from build123d import *

# Parameters (mm, degrees)
EXTRUDE_1_DEPTH             = 10
CUT_EXTRUDE_1_DEPTH         = 2
CUT_EXTRUDE_2_DEPTH         = 2
SKETCH_4_R                  = 35.00000000000001
CUT_EXTRUDE_3_DEPTH         = 3
CUT_EXTRUDE_4_DEPTH         = 62.016391240387215
HOLE_WIZARD_M3_1_D          = 2.5
HOLE_WIZARD_1_D             = 3.4
HOLE_WIZARD_1_CSINK_D       = 6.6
HOLE_WIZARD_1_CSINK_ANGLE   = 90
SKETCH_11_R                 = 4.000000000000005
SKETCH_11_R_2               = 3.999999999999999
SKETCH_11_R_3               = 4
CUT_EXTRUDE_5_DEPTH         = 1
CHAMFER_1_SIZE              = 10
EXTRUDE_2_DEPTH             = 14
EXTRUDE_2_DIRECTION_2_REACH = 63.628
SKETCH_13_R                 = 1.5000000000000009
SKETCH_13_R_2               = 1.5000000000000042
CUT_EXTRUDE_6_DEPTH         = 8
SKETCH_13_3_R               = 1.5000000000000009
SKETCH_13_3_R_2             = 1.5000000000000042
CUT_EXTRUDE_7_DEPTH         = 3
MIRROR_START                = 45.74011537
MIRROR_6_OUTLINE_R          = 1.5
MIRROR_6_DEPTH              = 5
CUT_EXTRUDE_8_DEPTH         = 83.20937791832523
FILLET_1_R                  = 3
FILLET_2_R                  = 3
FILLET_5_R                  = 3
CHAMFER_2_SIZE              = 0.5


# Read off the part's stored shape, not the designer's step: 镜向6
with BuildPart() as part:
    # 草图1 → 凸台-拉伸1 (new body)
    with BuildSketch(Plane(origin=(0, 0, 0), x_dir=(1, 0, 0), z_dir=(0, 1, 0))):
        Polygon((-43, 43), (42.999999999999986, 43), (43, -42.99999999999999), (-43, -42.99999999999999), align=None)
    extrude(amount=EXTRUDE_1_DEPTH)

    # 草图2 → 切除-拉伸1 (cut)
    with BuildSketch(Plane.XZ):
        Polygon((42.99999999999999, 7.000000000000008), (-43, 7.000000000000008), (-43, -43), (43, -43), align=None)
    extrude(amount=-CUT_EXTRUDE_1_DEPTH, mode=Mode.SUBTRACT)

    # 草图3 → 切除-拉伸2 (cut)
    with BuildSketch(Plane(origin=(0, 10, 0), x_dir=(1, 0, 0), z_dir=(0, 1, 0))):
        with BuildLine():
            Line((-24.686291501015234, -42.99999999999999), (24.686291501015248, -42.999999999999986))
            Line((24.686291501015244, -42.999999999999986), (24.686291501015237, -39.994837315919945))
            ThreePointArc((24.686291501015248, -39.99483731591996), (33.99829514057673, -32.45174768073728), (41.099999999999305, -22.79890348240587))
            Line((41.10000000000001, -22.798903482406033), (41.1, 22.798903482403997))
            ThreePointArc((41.10000000000031, 22.798903482404068), (33.23401871576778, 33.234018715767704), (22.79890348240416, 41.10000000000025))
            Line((22.798903482404093, 41.099999999999994), (-22.798903482403766, 41.099999999999994))
            ThreePointArc((-22.798903482403876, 41.1000000000004), (-33.23401871576702, 33.23401871576845), (-41.099999999999426, 22.798903482405624))
            Line((-41.1, 22.798903482405752), (-41.099999999999994, -22.798903482407027))
            ThreePointArc((-41.09999999999881, -22.798903482406732), (-33.99829514057638, -32.45174768073764), (-24.68629150101524, -39.99483731591995))
            Line((-24.686291501015234, -39.994837315919945), (-24.686291501015234, -42.99999999999999))
        make_face()
    extrude(amount=-CUT_EXTRUDE_2_DEPTH, mode=Mode.SUBTRACT)

    # 草图4 → 切除-拉伸3 (cut)
    with BuildSketch(Plane(origin=(0, 8, 0), x_dir=(1, 0, 0), z_dir=(0, 1, 0))):
        with Locations(Location((0, 0, 0), (0, 0, 270))):
            Circle(SKETCH_4_R)
    extrude(amount=-CUT_EXTRUDE_3_DEPTH, mode=Mode.SUBTRACT)

    # 草图5 → 切除-拉伸4 (cut, through all)
    with BuildSketch(Plane(origin=(0, 5, 0), x_dir=(1, 0, 0), z_dir=(0, 1, 0))):
        with BuildLine():
            Line((-4.999999999999996, 9.999999999999993), (-4.999999999999998, 34.64101615137756))
            ThreePointArc((-5, 34.64101615137755), (-22.872417196250915, 26.49249953478618), (-33.54101966249686, 9.999999999999986))
            Line((-33.54101966249684, 9.999999999999977), (-4.999999999999996, 9.999999999999993))
        make_face()
        with BuildLine():
            ThreePointArc((33.54101966249686, 9.999999999999986), (22.87241719625092, 26.492499534786173), (5.0000000000000036, 34.64101615137755))
            Line((5.000000000000002, 34.64101615137756), (5.000000000000006, 9.999999999999993))
            Line((5.000000000000006, 9.999999999999995), (33.54101966249686, 9.999999999999986))
        make_face()
        with BuildLine():
            Line((-4.99999999999999, -9.999999999999996), (-33.54101966249684, -9.999999999999995))
            ThreePointArc((-33.54101966249685, -9.999999999999993), (-22.87241719625092, -26.492499534786173), (-4.999999999999993, -34.64101615137755))
            Line((-4.999999999999981, -34.64101615137756), (-4.99999999999999, -9.999999999999996))
        make_face()
        with BuildLine():
            ThreePointArc((5.000000000000011, -34.64101615137755), (22.87241719625091, -26.49249953478618), (33.54101966249685, -9.999999999999991))
            Line((33.54101966249686, -9.999999999999986), (5.000000000000006, -9.999999999999995))
            Line((5.000000000000006, -9.999999999999993), (5.000000000000002, -34.64101615137756))
        make_face()
    extrude(amount=-CUT_EXTRUDE_4_DEPTH, mode=Mode.SUBTRACT)

    # M3 螺纹孔1 (through all)
    with Locations(Plane(origin=(0, 8, 0), x_dir=(1, 0, 0), z_dir=(0, 1, 0))):
        with Locations((-30.405591591, 30.405591591), (30.405591591, 30.405591591), (30.405591591, -30.405591591), (-30.405591591, -30.405591591)):
            Hole(HOLE_WIZARD_M3_1_D / 2)

    # 打孔尺寸(%根据十字)槽沉头木螺钉的类型1 (through all)
    with Locations(Plane(origin=(0, 8, 0), x_dir=(1, 0, 0), z_dir=(0, 1, 0))):
        with Locations((-33, 23), (33, 23), (0, 0)):
            CounterSinkHole(HOLE_WIZARD_1_D / 2, HOLE_WIZARD_1_CSINK_D / 2, counter_sink_angle=HOLE_WIZARD_1_CSINK_ANGLE)

    # 草图11 → 切除-拉伸5 (cut)
    with BuildSketch(Plane.XZ.offset(-2)):
        with Locations(Location((33, -23.000000000000007, 0), (0, 0, 270))):
            Circle(SKETCH_11_R)
        with Locations(Location((-33, -23, 0), (0, 0, 270))):
            Circle(SKETCH_11_R_2)
        with Locations(Location((0, 0, 0), (0, 0, 270))):
            Circle(SKETCH_11_R_3)
    extrude(amount=-CUT_EXTRUDE_5_DEPTH, mode=Mode.SUBTRACT)

    # 倒角1
    chamfer_1_edges = [part.edges().sort_by_distance(p)[0] for p in [
        (43, 5, 42.99999999999999),
        (-43, 5, 42.99999999999999),
        (-43, 6, -43),
        (42.999999999999986, 6, -43),
    ]]
    chamfer(chamfer_1_edges, length=CHAMFER_1_SIZE)

    # 草图12 → 凸台-拉伸2 (add)
    with BuildSketch(Plane(origin=(0, 10, 0), x_dir=(1, 0, 0), z_dir=(0, 1, 0))):
        Polygon((-21.68629150101517, -42.99999999999999), (-32.999999999999986, -42.99999999999999), (-10.171572875253744, -65.82842712474618), (10.171572875253764, -65.82842712474618), (32.999999999999986, -42.99999999999999), (21.68629150101517, -42.99999999999999), (4.514718625761375, -60.17157287525379), (-4.51471862576136, -60.17157287525379), align=None)
    extrude(amount=EXTRUDE_2_DEPTH)

    # 凸台-拉伸2 direction 2: up to this face of the body (flat: up to its plane)
    extrude_2_direction_2_end = Plane(part.part.faces().sort_by_distance((0, 0, 26.766223415))[0])
    # 草图12 → 凸台-拉伸2 direction 2 (add, up to the picked face)
    with BuildSketch(Plane(origin=(0, 10, 0), x_dir=(1, 0, 0), z_dir=(0, 1, 0)), mode=Mode.PRIVATE) as extrude_2_direction_2_sk1:
        Polygon((-21.68629150101517, -42.99999999999999), (-32.999999999999986, -42.99999999999999), (-10.171572875253744, -65.82842712474618), (10.171572875253764, -65.82842712474618), (32.999999999999986, -42.99999999999999), (21.68629150101517, -42.99999999999999), (4.514718625761375, -60.17157287525379), (-4.51471862576136, -60.17157287525379), align=None)
    extrude_2_direction_2_tool1 = split(extrude(extrude_2_direction_2_sk1.sketch, amount=-EXTRUDE_2_DIRECTION_2_REACH, mode=Mode.PRIVATE), bisect_by=extrude_2_direction_2_end, keep=Keep.BOTH, mode=Mode.PRIVATE)
    add(extrude_2_direction_2_tool1.solids().sort_by(Axis((-13.594324, 10, 52.079605), (0, -1, 0)))[0])

    # 草图13 → 切除-拉伸6 (cut)
    with BuildSketch(Plane(origin=(-38.00000000000007, 0, 37.999999999999886), x_dir=(0.7071067811865458, 0, 0.7071067811865492), z_dir=(-0.7071067811865492, 0, 0.7071067811865458))):
        with Locations((17.35533905932751, 20.999999999999993)):
            Circle(SKETCH_13_R)
        with Locations((34.35533905932751, 20.999999999999996)):
            Circle(SKETCH_13_R_2)
        with Locations((33.35533905932751, 11)):
            Circle(SKETCH_13_R_2)
        with Locations((18.35533905932751, 10.999999999999998)):
            Circle(SKETCH_13_R)
    extrude(amount=-CUT_EXTRUDE_6_DEPTH, mode=Mode.SUBTRACT)

    # 草图13<3> → 切除-拉伸7 (cut)
    with BuildSketch(Plane(origin=(-38.00000000000007, 0, 37.999999999999886), x_dir=(0.7071067811865458, 0, 0.7071067811865492), z_dir=(-0.7071067811865492, 0, 0.7071067811865458))):
        Polygon((38.35533905932751, 24), (13.355339059327509, 23.999999999999996), (13.355339059327513, 0), (38.35533905932752, 3.06e-15), align=None)
        with Locations((18.35533905932751, 10.999999999999998)):
            Circle(SKETCH_13_3_R, mode=Mode.SUBTRACT)
        with Locations((33.35533905932751, 11)):
            Circle(SKETCH_13_3_R_2, mode=Mode.SUBTRACT)
        with Locations((17.35533905932751, 20.999999999999993)):
            Circle(SKETCH_13_3_R, mode=Mode.SUBTRACT)
        with Locations((34.35533905932751, 20.999999999999996)):
            Circle(SKETCH_13_3_R_2, mode=Mode.SUBTRACT)
    extrude(amount=-CUT_EXTRUDE_7_DEPTH, mode=Mode.SUBTRACT)

    # 镜向6 outline → 镜向6 (cut)
    with BuildSketch(Plane(origin=(0, 0, 0), x_dir=(0.707106781186546, 0, -0.707106781186549), z_dir=(0.707106781186549, 0, 0.707106781186546)).offset(MIRROR_START)):
        with Locations((-17.355339059, 21)):
            Circle(MIRROR_6_OUTLINE_R)
        with Locations((-18.355339059, 11)):
            Circle(MIRROR_6_OUTLINE_R)
        with Locations((-33.355339059, 11)):
            Circle(MIRROR_6_OUTLINE_R)
        with Locations((-34.355339059, 21)):
            Circle(MIRROR_6_OUTLINE_R)
    extrude(amount=MIRROR_6_DEPTH, mode=Mode.SUBTRACT)

    # 草图14 → 切除-拉伸8 (cut, through all)
    with BuildSketch(Plane(origin=(0, 24, 0), x_dir=(1, 0, 0), z_dir=(0, 1, 0))):
        Polygon((-2e-17, -65.82842712474616), (-1e-17, -63.00000000000004), (-8.757359312880741, -63.00000000000004), (-10.878679656440386, -65.12132034355969), (-10.171572875253748, -65.82842712474616), align=None)
        Polygon((8.757359312880741, -63.00000000000004), (0, -63.00000000000004), (-2e-17, -65.82842712474616), (10.171572875253762, -65.82842712474618), (10.878679656440323, -65.12132034355963), align=None)
        Polygon((26.435028842544384, -45.32233047033632), (8.757359312880741, -63.00000000000004), (10.878679656440386, -65.12132034355969), (28.556349186104022, -47.44365081389593), align=None)
    extrude(amount=-CUT_EXTRUDE_8_DEPTH, mode=Mode.SUBTRACT)

    # 圆角1
    fillet_1_edges = [part.edges().sort_by_distance(p)[0] for p in [
        (42.99999999999999, 1, 7.000000000000008),
        (-43, 1, 7.000000000000008),
        (33.54101966249685, 2.5, 9.99999999999999),
        (5.000000000000006, 2.5, 9.999999999999993),
        (5.000000000000007, 2.5, 34.641016151377556),
        (-4.999999999999988, 2.5, 34.641016151377556),
        (-4.99999999999999, 2.5, 9.999999999999996),
        (-33.54101966249685, 2.5, 9.999999999999993),
        (33.541019662496865, 3.5, -9.999999999999988),
        (5.000000000000006, 3.5, -9.999999999999993),
        (5.0000000000000036, 3.5, -34.641016151377556),
        (-5, 3.5, -34.641016151377556),
        (-4.999999999999996, 3.5, -9.999999999999993),
        (-33.54101966249685, 3.5, -9.999999999999982),
        (-41.0999999999994, 9, 22.798903482406878),
        (-41.09999999999971, 9, -22.798903482405688),
        (41.10000000000016, 9, -22.798903482404036),
        (41.09999999999966, 9, 22.798903482405954),
        (-22.798903482403823, 9, -41.1000000000002),
        (22.798903482404132, 9, -41.10000000000012),
        (24.686291501015248, 9, 42.999999999999986),
        (-24.686291501015234, 9, 42.99999999999999),
    ]]
    fillet(fillet_1_edges, radius=FILLET_1_R - 0.0001)  # a hair under: the kernel refuses the full size

    # 圆角2
    fillet_2_edges = [part.edges().sort_by_distance(p)[0] for p in [
        (27.34319575050762, 10, 42.99999999999999),
        (-27.34319575050762, 10, 42.99999999999999),
    ]]
    fillet(fillet_2_edges, radius=FILLET_2_R - 0.0001)  # a hair under: the kernel refuses the full size

    # 圆角5
    fillet_5_edges = [part.edges().sort_by_distance(p)[0] for p in [
        (21.68629150101517, 4, 42.99999999999999),
        (-21.68629150101517, 4, 42.99999999999999),
        (-4.514718625761361, 12, 60.17157287525379),
        (4.514718625761375, 12, 60.17157287525379),
    ]]
    fillet(fillet_5_edges, radius=FILLET_5_R)

    # 倒角2
    chamfer_2_edges = [part.edges().sort_by_distance(p)[0] for p in [
        (-28.556349186104043, 11.999999999999998, 47.44365081389596),
        (28.55634918610403, 11.999999999999998, 47.44365081389594),
    ]]
    chamfer(chamfer_2_edges, length=CHAMFER_2_SIZE)


solid = part.part
The listing builds one solid part. Answer for the finished solid, in the listing's coordinates (mm). A direction names the side the tool comes from. Give positions to 0.01 mm unless a question says otherwise; leave off trailing zeros. Order: outer loops, then holes, each group sorted by start corner. A loop starts at its lowest first (then second) coordinate and runs counter-clockwise, first axis right, second up. Notation, with made-up numbers: (84, 70) -> (119, 70) arc R26 cw to (119, 109) -> close; hole circle Ø3 at (-13.5, 17.5). An arc over 180 degrees is marked (long way). Put each result on its own line as item: value.
Item 1: For a pull along Y with two mould halves and no side action, classify faces 4 (the face through (18, 4, -10)), 5 (the face through (-21.295, 12.487, 46.977)), 6 (the face through (0, 10, -42)) as released by +Y, released by -Y, zero draft, split by the parting line, or undercut.
Established:
face 4: zero draft
face 5: undercut
face 6: released by +Y
Item 2: A cutting plane is placed at A-A on x = 0. Give the vertices of the cut face in (y, z).
Established:
outline: (0, 7) -> (2, 7) -> (2, 4) -> (3, 4) -> (3, 1.7) -> (5, 1.7) -> (5, 35) -> (8, 35) -> (8, 43) -> (0, 43) -> close; (0, 60.17) -> (24, 60.17) -> (24, 63) -> (0, 63) -> close; (2, -43) -> (10, -43) -> (10, -41.1) -> (8, -41.1) -> (8, -35) -> (5, -35) -> (5, -1.7) -> (3, -1.7) -> (3, -4) -> (2, -4) -> close
Item 3: For faces 1 (the face through (13.654, 11.832, 51.032)), 2 (the face through (-17.196, 3.944, 44.806)), 3 (the face through (-28.94, 10.9, 42.14)), determine the directions among +Z, -Z, +X, -X, +Y, -Y from which every point of the face is accessible in a straight line to the end or side of a thin tool.
Established:
face 1: +Y
face 2: +Y, -Y
face 3: -Z, +X, -X, +Y
Item 4: Given P1, Ø10, axis at x = -23.5, y = 19.5, coming from the -Z side; P2, Ø6.5, axis at x = 0, z = 1.5, coming from the -Y side; P3, Ø7, axis at x = 0, z = 0, coming from the +Y side, each flat-ended and moving along its own axis, determine where each tip first touches the part or whether it passes through.
Established:
P1: stops at z = 43
P2: stops at y = 2
P3: stops at y = 5
Item 5: A cutting plane is placed at B-B on z = 0. Give the vertices of the cut face in (x, y), plus the area to 3 significant figures.
Established:
outline: (-43, 2) -> (-4, 2) -> (-4, 3) -> (-1.7, 3) -> (-1.7, 5) -> (-35, 5) -> (-35, 8) -> (-41.1, 8) -> (-41.1, 10) -> (-43, 10) -> close; (1.7, 3) -> (4, 3) -> (4, 2) -> (43, 2) -> (43, 10) -> (41.1, 10) -> (41.1, 8) -> (35, 8) -> (35, 5) -> (1.7, 5) -> close
area: 299 mm^2
Item 6: Straight lines are drawn through the part: line 1 (Z direction, x = 0, y = 5.5); line 2 (Z direction, x = 3, y = 2.5); line 3 (X direction, y = 5.5, z = -23). For each, find the intervals that lie inside material, in ascending order.
Established:
line 1: z = -43 to -35, 35 to 43, 60.17 to 63
line 2: z = -43 to -2.65, 2.65 to 43, 60.17 to 63
line 3: x = -43 to -34.7, -31.3 to -26.38, 26.38 to 31.3, 34.7 to 43
